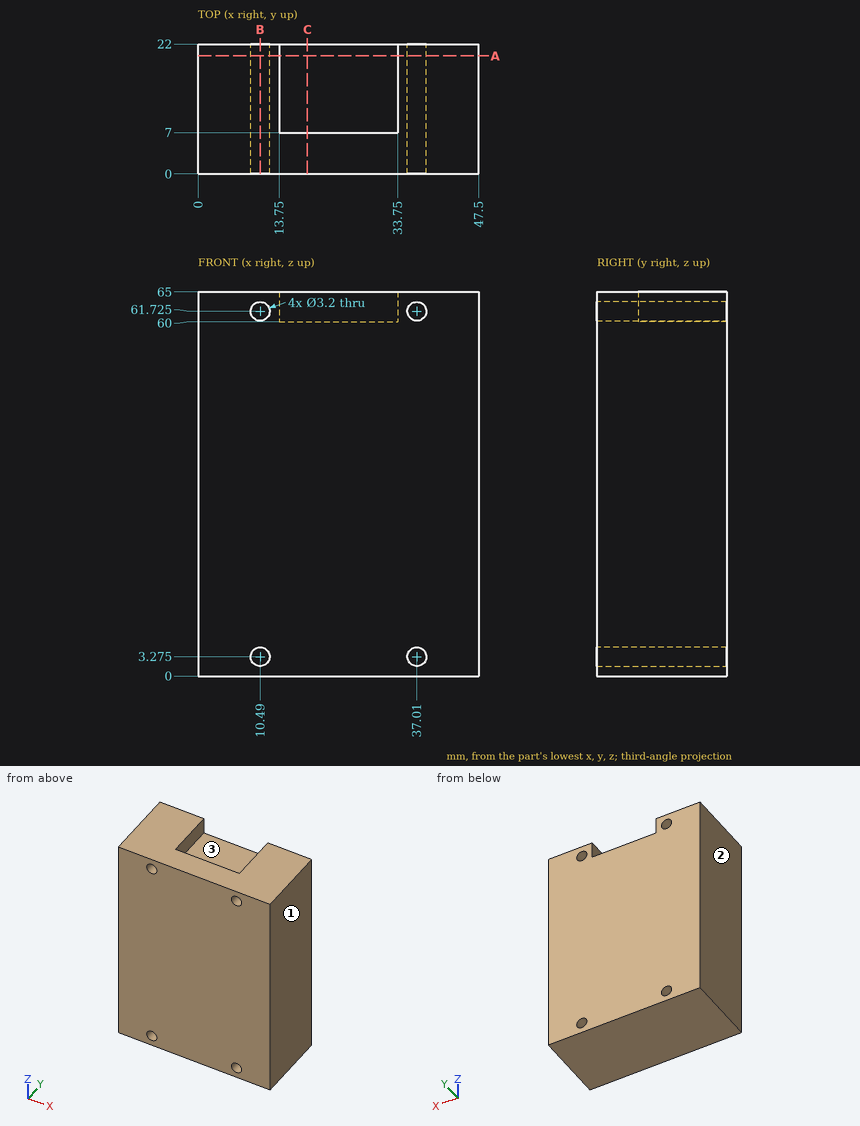
Can you work these out from the drawing? Everything is in mm from the part's minimum corner. Give positions to 0.01 mm unless a question says otherwise; leave off trailing zeros. Loops run counter-clockwise (first coordinate to the right, second up) from the corner with the lowest first, then second, coordinate; pieces in that order, holes last. Notation, with made-up numbers: (44, -23.75) -> (54, -23.75) arc R12 cw to (54, -11.75) -> close; hole circle Ø2 at (-23, 76). An arc over 180 degrees is marked (long way). Write item = value, one per line.
1) Will this pin go through, and if not, where does the flat tip stop? pin 1 (4 mm diameter, centred on x = 19, z = 63.5, fed in from +Y).
Check result:
pin_1 = 7
2) I need wall thicknesses on L1, parallel to Z at x = 37.5, y = 6; L2, parallel to X at y = 9.75, z = 4; L3, parallel to Z at x = 36, y = 13.25. Which ranges of each line are inside material? Lowest first, please. Write a range as from..to.
Check result:
L1 = 0..1.75, 4.8..60.2, 63.25..65
L2 = 0..9.06, 11.92..35.58, 38.44..47.5
L3 = 0..2.03, 4.52..60.48, 62.97..65
3) Thinking about a two-plate mould opening in X: for the marked faces 1, 2 and 3, which applies, released by +X, released by -X, zero draft, split by the parting line, or undercut?
Check result:
face_1 = released by +X
face_2 = released by -X
face_3 = undercut
4) Suppose I cut it at A-A on y = 20. Write out the boundary of the cut face in (x, z) (3 decimals).
Check result:
outline = (0, 0) -> (47.5, 0) -> (47.5, 65) -> (33.75, 65) -> (33.75, 60) -> (13.75, 60) -> (13.75, 65) -> (0, 65) -> close; hole circle Ø3.2 at (10.49, 3.275); hole circle Ø3.2 at (10.49, 61.725); hole circle Ø3.2 at (37.01, 3.275); hole circle Ø3.2 at (37.01, 61.725)
5) Suppose I cut it at B-B on x = 10.49. Write out the boundary of the cut face in (y, z) (3 decimals).
Check result:
outline = (0, 0) -> (22, 0) -> (22, 1.675) -> (0, 1.675) -> close; (0, 4.875) -> (22, 4.875) -> (22, 60.125) -> (0, 60.125) -> close; (0, 63.325) -> (22, 63.325) -> (22, 65) -> (0, 65) -> close
6) Suppose I cut it at C-C on x = 18.5. Write out the boundary of the cut face in (y, z).
Check result:
outline = (0, 0) -> (22, 0) -> (22, 60) -> (7, 60) -> (7, 65) -> (0, 65) -> close
